The listing builds one solid part. Answer for the finished solid, in the listing's coordinates (mm). A direction names the side the tool comes from. Coordinates: 2 decimals unless noted, no trailing zeros. Write each loop counter-clockwise with the first axis right and the second up, starting at its lowest first coordinate (ties: lowest second). Pieces come first, ordered by that corner, then holes. Notation, with made-up numbers: M 0.5,67.5 L 22.5,67.5 A24 cw 22.5,92.5 Z; hole C 18,-24 d9. An arc over 180 degrees is marked long. Answer as a JSON object with one key per item and string values. Group by question number.
from build123d import *

# Parameters (mm, degrees)
F0_W          = 76.2
F0_H          = 101.6
F0_R          = 19.05
F1_DEPTH      = 152.4
F2_R          = 22.225
F3_DEPTH      = 38.101
F3_DEPTH_BACK = 139.23277
F5_DEPTH      = 101.601


with BuildPart() as f1:
    # F0 (on Front) → F1 (new body, symmetric)
    with BuildSketch(Plane.XZ):
        Rectangle(F0_W, F0_H)
        Circle(F0_R, mode=Mode.SUBTRACT)
    extrude(amount=F1_DEPTH, both=True)

    # F2 (on Right) → F3 (cut, two sides)
    with BuildSketch(Plane.YZ) as f3_sk:
        Circle(F2_R)
    extrude(amount=F3_DEPTH, mode=Mode.SUBTRACT)
    extrude(f3_sk.sketch, amount=-F3_DEPTH_BACK, mode=Mode.SUBTRACT)

    # F4 (on face) → F5 (cut, through all)
    with BuildSketch(Plane.XY.offset(50.8)):
        Polygon((9.525, -97.802216), (-9.525, -97.802216), (-19.05, -114.3), (-9.525, -130.797784), (9.525, -130.797784), (19.05, -114.3), align=None)
    extrude(amount=-F5_DEPTH, mode=Mode.SUBTRACT)


solid = f1.part
Item 1: For a pull along Z with two mould halves and no side action, classify faces 3 (the face through (-14.041, -137.317, 12.875)), 4 (the face through (-1, -2, -50.8)), 5 (the face through (16, -152.4, 12)) as +Z half, -Z half, draft (parallel to the pull), parting line (faces both ways), or undercut.
Item 2: A cutting plane is placed at C-C, the plane z = -12. Write down the section's boundary in (x, y).
Item 3: A flat-ended cylindrical pin translates along its axis: pin 1 Ø10 at (x, z) = (14.5, -8) entering from -Y. Find the tip coordinate at first contact, or state that the pin passes through.
Item 4: A cutting plane is placed at A-A, the plane x = 0. Write down the section's boundary in (y, z) (3 decimals), and give its area (3 significant figures).
Item 5: A cutting plane is placed at D-D, the plane z = -42. Write down the section's boundary in (x, y) (3 decimals), and give its area (3 significant figures).
Item 6: A cutting plane is placed at B-B, the plane y = 0. Write down the section's boundary in (x, z) (3 decimals).
Item 7: A tool of negligible diameter and unlimited length cuts with its end or side. For faces 1 (the face through (-19.03, 82.91, 0.84)), 2 (the face through (14.354, -106.167, -30.689)), from which of +Z, -Z, +X, -X, +Y, -Y can it reach the whole face along a straight path? Write none if from no direction.
Item 8: Consider L1, parallel to X at y = 115, z = 0; L2, parallel to Z at x = 0, y = -139; L3, parallel to Y at x = -19, z = -6. Determine where each line is inside the solid, lowest interval first. Write a range as from..to.
Answer:
{
 "1": {"face 3": "undercut", "face 4": "-Z half", "face 5": "draft"},
 "2": {"outline": "M -38.1,-152.4 L -14.8,-152.4 L -14.8,-121.67 L -19.05,-114.3 L -14.8,-106.93 L -14.8,-18.71 L -38.1,-18.71 Z; M -38.1,18.71 L -14.8,18.71 L -14.8,152.4 L -38.1,152.4 Z; M 14.8,-152.4 L 38.1,-152.4 L 38.1,-18.71 L 14.8,-18.71 L 14.8,-106.93 L 19.05,-114.3 L 14.8,-121.67 Z; M 14.8,18.71 L 38.1,18.71 L 38.1,152.4 L 14.8,152.4 Z"},
 "3": {"pin 1": "y = -152.4"},
 "4": {"outline": "M -152.4,-50.8 L -130.798,-50.8 L -130.798,-19.05 L -152.4,-19.05 Z; M -152.4,19.05 L -130.798,19.05 L -130.798,50.8 L -152.4,50.8 Z; M -97.802,-50.8 L 152.4,-50.8 L 152.4,-19.05 L 11.448,-19.05 A22.225 cw -11.448,-19.05 L -97.802,-19.05 Z; M -97.802,19.05 L -11.448,19.05 A22.225 cw 11.448,19.05 L 152.4,19.05 L 152.4,50.8 L -97.802,50.8 Z", "area": "17,200 mm2"},
 "5": {"outline": "M -38.1,-152.4 L 38.1,-152.4 L 38.1,152.4 L -38.1,152.4 Z; hole M -19.05,-114.3 L -9.525,-130.798 L 9.525,-130.798 L 19.05,-114.3 L 9.525,-97.802 L -9.525,-97.802 Z", "area": "22,300 mm2"},
 "6": {"outline": "M -38.1,-50.8 L 38.1,-50.8 L 38.1,-22.225 L -38.1,-22.225 Z; M -38.1,22.225 L 38.1,22.225 L 38.1,50.8 L -38.1,50.8 Z"},
 "7": {"face 1": "+Y, -Y", "face 2": "+Z, -Z"},
 "8": {"L1": "-38.1..-19.05, 19.05..38.1", "L2": "-50.8..-19.05, 19.05..50.8", "L3": "-152.4..-114.39, -114.21..-21.4, 21.4..152.4"}
}
